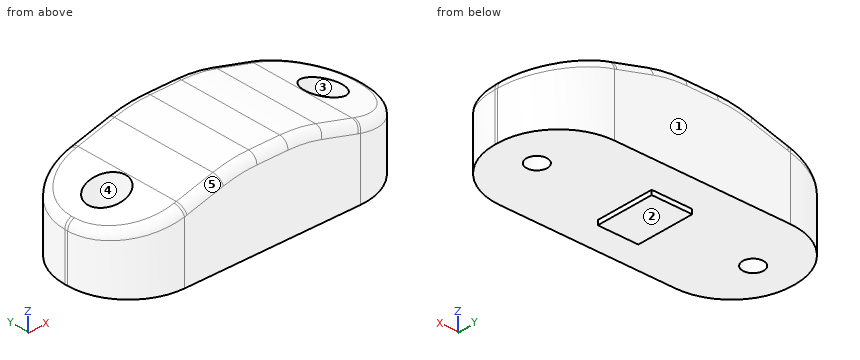
```python
from build123d import *

# Parameters (mm, degrees)
SKETCH1_R           = 2.3
BOSS_EXTRUDE1_DEPTH = 19
CUT_EXTRUDE1_DEPTH  = 48.088108902
FILLET1_R           = 30
FILLET2_R           = 2
SKETCH3_R           = 4.2
CUT_EXTRUDE2_DEPTH  = 11
SKETCH4_W           = 9
SKETCH4_H           = 13
BOSS_EXTRUDE2_DEPTH = 1


with BuildPart() as part:
    # Sketch1 → Boss-Extrude1 (new body)
    with BuildSketch(Plane.XY):
        with BuildLine():
            Line((-19.5, 13.85), (19.5, 13.85))
            ThreePointArc((19.5, 13.85), (29.045941546, 9.895941546), (33, 0.35))
            Line((33, 0.35), (33, -0.35))
            ThreePointArc((33, -0.35), (29.045941546, -9.895941546), (19.5, -13.85))
            Line((19.5, -13.85), (-19.5, -13.85))
            ThreePointArc((-19.5, -13.85), (-29.045941546, -9.895941546), (-33, -0.35))
            Line((-33, -0.35), (-33, 0.35))
            ThreePointArc((-33, 0.35), (-29.045941546, 9.895941546), (-19.5, 13.85))
        make_face()
        with Locations((-24, 0)):
            Circle(SKETCH1_R, mode=Mode.SUBTRACT)
        with Locations((24, 0)):
            Circle(SKETCH1_R, mode=Mode.SUBTRACT)
    extrude(amount=BOSS_EXTRUDE1_DEPTH)

    # Sketch2 → Cut-Extrude1 (cut, through all)
    with BuildSketch(Plane.XZ.offset(13.85)):
        Polygon((-19.5, 19), (-19.5, 15.705882353), (-7.5, 19), align=None)
        Polygon((-33, 12), (-19.5, 15.705882353), (-19.5, 19), (-33, 19), align=None)
        Polygon((7.5, 19), (19.5, 15.705882353), (19.5, 19), align=None)
        Polygon((19.5, 19), (19.5, 15.705882353), (33, 12), (33, 19), align=None)
    extrude(amount=-CUT_EXTRUDE1_DEPTH, mode=Mode.SUBTRACT)

    # Fillet1
    fillet1_edges = [part.edges().sort_by_distance(p)[0] for p in [
        (-7.5, 0, 19),
        (7.5, 0, 19),
    ]]
    fillet(fillet1_edges, radius=FILLET1_R)

    # Fillet2
    fillet2_edges = [part.edges().sort_by_distance(p)[0] for p in [
        (-33, 0, 12),
        (-15.449321203, -13.85, 16.817833395),
        (-28.958901568, 9.982195032, 13.109321138),
        (-15.449321203, 13.85, 16.817833395),
        (-28.958901568, -9.982195032, 13.109321138),
        (33, 0, 12),
        (15.449321203, -13.85, 16.817833395),
        (28.958901568, 9.982195032, 13.109321138),
        (28.958901568, -9.982195032, 13.109321138),
        (15.449321203, 13.85, 16.817833395),
        (0, -13.85, 19),
        (-7.463781607, -13.85, 18.731242264),
        (7.463781607, -13.85, 18.731242264),
        (0, 13.85, 19),
        (-7.463781607, 13.85, 18.731242264),
        (7.463781607, 13.85, 18.731242264),
    ]]
    fillet(fillet2_edges, radius=FILLET2_R)

    # Sketch3 → Cut-Extrude2 (cut)
    with BuildSketch(Plane.XY.offset(19)):
        with Locations((-24, 0)):
            Circle(SKETCH3_R)
        with Locations(Location((24, 0, 0), (0, 0, 180))):
            Circle(SKETCH3_R)
    extrude(amount=-CUT_EXTRUDE2_DEPTH, mode=Mode.SUBTRACT)

    # Sketch4 → Boss-Extrude2 (add)
    with BuildSketch(Plane(origin=(0, 0, 0), x_dir=(-1, 0, 0), z_dir=(0, 0, -1))):
        Rectangle(SKETCH4_W, SKETCH4_H)
    extrude(amount=BOSS_EXTRUDE2_DEPTH)


solid = part.part
```
Geometry check sheet. Reference: the model listing, model coordinates, mm. Face numbers are marked on the shaded views. A direction names the side the tool comes from. Coordinates: 2 decimals unless noted, no trailing zeros. Write each loop counter-clockwise with the first axis right and the second up, starting at its lowest first coordinate (ties: lowest second). Pieces come first, ordered by that corner, then holes. Notation, with made-up numbers: M 83.25,56 L 115.25,56 A22 ccw 115.25,78 Z; hole C -9,58.25 d9. An arc over 180 degrees is marked long. Answer as a JSON object with one key per item and string values.
1. Scan lines: L1, parallel to X at y = 0, z = 2; L2, parallel to X at y = -1, z = 5.75; L3, parallel to Z at x = 27, y = 4.5. Record each from-to range of solid material in increasing order.
Answers below:
{"L1": "x = -33 to -26.3, -21.7 to 21.7, 26.3 to 33", "L2": "x = -32.98 to -26.07, -21.93 to 21.93, 26.07 to 32.98", "L3": "z = 0 to 13.65"}
2. Tool access check on the marked faces 4 and 5. Record the directions out of +Z, -Z, +X, -X, +Y, -Y that give a thin tool (end or side, any length) a straight path to the whole face; none if there is none.
Answers below:
{"face 4": "+Z", "face 5": "+Z, -X, -Y"}
3. Go/stop test with flat-tipped pins: pin 1 Ø6 at (x, y) = (24, 0) entering from +Z; pin 2 Ø5 at (x, y) = (-4.5, -9.5) entering from -Z; pin 3 Ø3 at (y, z) = (-10.5, 13.5) entering from +X; pin 4 Ø1.1 at (x, z) = (-1.5, -0.5) entering from +Y. Record where each tip stops, or that it passes through.
Answers below:
{"pin 1": "stops at z = 8", "pin 2": "stops at z = 0", "pin 3": "stops at x = 29.05", "pin 4": "stops at y = 13.85"}
4. Section check B-B, the plane z = 13. Give the number of separate pieces and of enclosed holes in the cut face, plus the area to 3 significant figures.
Answers below:
{"separate pieces": "1", "enclosed holes": "2", "area": "1,450 mm²"}
5. Draft check along Y on the marked faces 1, 2 and 3. Enter one of: released by +Y, released by -Y, zero draft, split by the parting line, or undercut.
Answers below:
{"face 1": "released by +Y", "face 2": "zero draft", "face 3": "undercut"}
6. Section check A-A, the plane z = 5. Enter the section's corners in (x, y).
Answers below:
{"outline": "M -33,-0.35 A13.5 ccw -19.5,-13.85 L 19.5,-13.85 A13.5 ccw 33,-0.35 L 33,0.35 A13.5 ccw 19.5,13.85 L -19.5,13.85 A13.5 ccw -33,0.35 Z; hole C -24,0 d4.6; hole C 24,0 d4.6"}
